from build123d import *

# Parameters (mm, degrees)
F2_W     = 5.632173
F2_H     = 2.54
F3_DEPTH = 25.4


with BuildPart() as f1:
    # F0 (on Front) → F1 (revolve)
    with BuildSketch(Plane.XZ):
        Polygon((-9.306035, 0), (0, 0), (0, 3.175), (-7.434009, 3.175), (-17.411153, 22.59206), (-20.914602, 22.59206), align=None)
    revolve(axis=Axis((0, 0, 1.5875), (0, 0, -1)))

    # F2 (on face) → F3 (cut)
    with BuildSketch(Plane.XY.offset(3.175)):
        with Locations((0.276086, 0)):
            Rectangle(F2_W, F2_H)
    extrude(amount=-F3_DEPTH, mode=Mode.SUBTRACT)


solid = f1.part
Geometry check sheet. Reference: the model listing, model coordinates, mm. A direction names the side the tool comes from. Give positions to 0.01 mm unless a question says otherwise; leave off trailing zeros. Loops run counter-clockwise (first coordinate to the right, second up) from the corner with the lowest first, then second, coordinate; pieces in that order, holes last. Notation, with made-up numbers: M -22.5,60.5 L 26.5,60.5 A24 ccw 26.5,91.5 Z; hole C 24.25,63.25 d10. An arc over 180 degrees is marked long. Answer as a JSON object with one key per item and string values. Group by question number.
Item 1: Sectioned sample at D-D on z = 7.75. Record the boundary of the cut face in (x, y).
Item 2: Mould release check, pull along X, two halves, no side actions. Record for faces 4 (the flat face through (-8, 16, 22.592)), 5 (the conical face through (-11.874, 3.739, 6.117)), 6 (the flat face through (3.092, 0, 2)): pulls with the +X half, pulls with the -X half, needs draft (parallel to the pull), parting line crosses it, or undercut.
Item 3: Access from +Z, -Z, +X, -X, +Y, -Y to the whole of each face (thin tool, end or side, straight path). Record for faces 1 (the flat face through (0, -2, 0)), 2 (the flat face through (0, -1.27, 2)), 3 (the flat face through (0, -2, 3.175)).
Item 4: Gauge pin test, flat ends, axial feed: pin 1 (2 mm diameter, centred on y = 0, z = 1.5, fed in from +X); pin 2 (2 mm diameter, centred on y = -0.5, z = 1, fed in from -X); pin 3 (1.6 mm diameter, centred on x = -1, z = 2, fed in from +Y). Record the tip position at first contact, or that the pin passes through.
Item 5: Sectioned sample at C-C on z = 14.5. Record the boundary of the cut face in (x, y).
Item 6: Sectioned sample at B-B on x = 0. Record the boundary of the cut face in (y, z) (3 decimals), plus the area to 3 significant figures.
Item 7: Sectioned sample at A-A on y = 0. Record the boundary of the cut face in (x, z) (3 decimals).
Item 8: Material ranges on L1, parallel to Y at x = -1, z = 2; L2, parallel to X at y = 0.5, z = 7.75; L3, parallel to X at y = 12, z = 20, recorded low to high.
Findings below:
{
 "1": {"outline": "C 0,0 d26.58; hole C 0,0 d19.57"},
 "2": {"face 4": "needs draft", "face 5": "parting line crosses it", "face 6": "undercut"},
 "3": {"face 1": "-Z, +X, -X, +Y, -Y", "face 2": "+Z, -Z", "face 3": "+Z"},
 "4": {"pin 1": "x = 10.59", "pin 2": "x = -10.32", "pin 3": "y = 10.7"},
 "5": {"outline": "C 0,0 d33.51; hole C 0,0 d26.51"},
 "6": {"outline": "M -20.915,22.592 L -9.306,0 L -1.27,0 L -1.27,3.175 L -7.434,3.175 L -17.411,22.592 Z; M 1.27,0 L 9.306,0 L 20.915,22.592 L 17.411,22.592 L 7.434,3.175 L 1.27,3.175 Z", "area": "192 mm2"},
 "7": {"outline": "M -20.915,22.592 L -9.306,0 L -2.54,0 L -2.54,3.175 L -7.434,3.175 L -17.411,22.592 Z; M 3.092,0 L 9.306,0 L 20.915,22.592 L 17.411,22.592 L 7.434,3.175 L 3.092,3.175 Z"},
 "8": {"L1": "-10.29 to -1.27, 1.27 to 10.29", "L2": "-13.28 to -9.77, 9.77 to 13.28", "L3": "-15.48 to -10.7, 10.7 to 15.48"}
}
